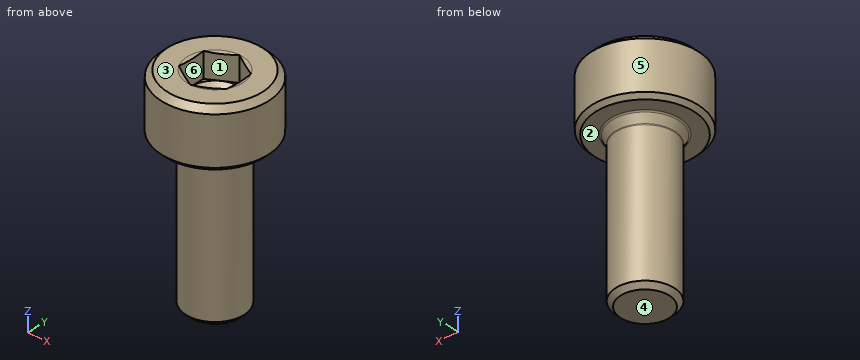
```python
from build123d import *

# Parameters (mm, degrees)
CUT_EXTRUDE1_DEPTH = 1.3


with BuildPart() as part:
    # Sketch1 → Revolve1 (revolve)
    with BuildSketch(Plane(origin=(0, 0, 0), x_dir=(0, 0, -1), z_dir=(1, 0, 0))):
        with BuildLine():
            Line((0, 0), (0, 2.45))
            Line((0, 2.45), (0.3, 2.75))
            Line((0.3, 2.75), (2.785, 2.75))
            Line((2.785, 2.75), (3, 2.535))
            Line((3, 2.535), (3, 1.8))
            ThreePointArc((3, 1.8), (3.015193643, 1.74701055), (3.056157637, 1.710123155))
            Line((3.056157637, 1.710123155), (3.466157637, 1.510123155))
            ThreePointArc((3.466157637, 1.510123155), (3.48750205, 1.50256365), (3.51, 1.5))
            Line((3.51, 1.5), (10.75, 1.5))
            Line((10.75, 1.5), (11, 1.25))
            Line((11, 1.25), (11, 0))
            Line((11, 0), (0, 0))
        make_face()
    revolve(axis=Axis((0, 0, 0), (0, 0, -1)))

    # Sketch2 → Cut-Extrude1 (cut)
    with BuildSketch(Plane.XY):
        Polygon((0, 1.443375673), (-1.25, 0.721687836), (-1.25, -0.721687836), (0, -1.443375673), (1.25, -0.721687836), (1.25, 0.721687836), align=None)
    extrude(amount=-CUT_EXTRUDE1_DEPTH, mode=Mode.SUBTRACT)

    # Sketch3 → Cut-Revolve2 (revolve, cut)
    with BuildSketch(Plane(origin=(0, 0, 0), x_dir=(0, 0, -1), z_dir=(1, 0, 0))):
        Polygon((1.3, 0), (1.3, 1.25), (2.021687836, 0), align=None)
    revolve(axis=Axis((0, 0, -1.3), (0, 0, -1)), mode=Mode.SUBTRACT)

    # Sketch4 → Cut-Revolve3 (revolve, cut)
    with BuildSketch(Plane(origin=(0, 0, 0), x_dir=(0, 0, -1), z_dir=(1, 0, 0))):
        Polygon((0, 1.443375673), (0, 1.25), (0.051814855, 1.25), align=None)
    revolve(axis=Axis((0, 0, 0), (0, 0, -1)), mode=Mode.SUBTRACT)


solid = part.part
```
CAD build for the part. Positions are in the model's coordinates, mm. Face numbers are marked on the shaded views. A direction names the side the tool comes from. Round coordinates to 2 decimals unless told otherwise and drop trailing zeros. Order: outer loops, then holes, each group sorted by start corner. A loop starts at its lowest first (then second) coordinate and runs counter-clockwise, first axis right, second up.
Q1. Slice it at B-B (z = -10). Write the cut outline in (x, y), and give its area (3 significant figures).
Q2. Two-plate mould, pull along X, no slides. Class the marked faces 4, 5 and 6: pulls with the +X half, pulls with the -X half, needs draft (parallel to the pull), parting line crosses it, or undercut.
Q3. Which spindle directions (+Z, -Z, +X, -X, +Y, -Y) get a long thin tool onto all of the face, cutting with end or side? Do the marked faces 1, 2 and 3. Say none if no direction does.
Q4. Slice it at A-A (z = -1). Write the cut outline in (x, y), and give its area (3 significant figures).
Q5. Drop flat-ended pins along their axis: pin 1 (1 mm diameter, centred on x = -1.5, y = -1, fed in from -Z); pin 2 (3 mm diameter, centred on y = 1, z = -5.5, fed in from +X); pin 3 (3 mm diameter, centred on x = 2, z = -6, fed in from +Y). Give the stop position or say it passes through.
Q6. Wall check: L1, parallel to Z at x = -0.7, y = -2; L2, parallel to Y at x = 0.1, z = -9; L3, parallel to X at y = 0.7, z = -3.25. Give the ranges that are in metal, low to high.
Results below:
1. outline: circle Ø3 at (0, 0)
1. area: 7.07 mm2
2. face 4: needs draft
2. face 5: parting line crosses it
2. face 6: undercut
3. face 1: +Z
3. face 2: -Z
3. face 3: +Z, +X, -X, +Y, -Y
4. outline: circle Ø5.5 at (0, 0); hole (-1.25, -0.72) - (0, -1.44) - (1.25, -0.72) - (1.25, 0.72) - (0, 1.44) - (-1.25, 0.72) - close
4. area: 18.3 mm2
5. pin 1: stops at z = -10.95
5. pin 2: stops at x = 1.5
5. pin 3: stops at y = 1.41
6. L1: z = -3 to 0
6. L2: y = -1.5 to 1.5
6. L3: x = -1.46 to 1.46
